Input: part model. Units: mm. Frame: model coordinates. Face numbers are marked on the shaded views. A direction names the side the tool comes from. Round coordinates to 2 decimals unless told otherwise and drop trailing zeros. Order: outer loops, then holes, each group sorted by start corner. A loop starts at its lowest first (then second) coordinate and runs counter-clockwise, first axis right, second up.
Item 1: Line query: L1, parallel to X at y = 12, z = -32; L2, parallel to Z at x = 20, y = 5.5; L3, parallel to Z at x = 37, y = 15. Output: solid intervals per line, ascending.
Item 2: Cut plane A-A on z = -32. Give the number of separate pieces and of enclosed holes in the cut face, then the cut area to 3 significant figures.
Item 3: Cut plane C-C on x = 20. Output: boundary loops of the cut face in (y, z).
Item 4: Cut plane D-D on z = -21. Output: boundary loops of the cut face in (x, y).
Item 5: Reachability of the marked faces 1, 2, 3 and 4 from +Z, -Z, +X, -X, +Y, -Y: full face, straight path, thin tool, end or side. Return the list, or none.
Item 6: Mould query, pull axis X, two halves, no side actions, for the marked faces 5, 6 and 7. Classes: released by +X, released by -X, zero draft, split by the parting line, or undercut.
Item 7: Cut plane B-B on y = 7.25. Output: boundary loops of the cut face in (x, z), then the cut area to 3 significant figures.
Item 8: First-contact query: pin 1 (5 mm diameter, centred on x = 4.5, z = -32, fed in from +Y); pin 2 (1 mm diameter, centred on y = 26.5, z = -12, fed in from +X); pin 3 (3.5 mm diameter, centred on y = 24, z = -7, fed in from -X). Flat tips, straight axial feed; report the tip coordinate or a pass-through.
```python
from build123d import *

# Parameters (mm, degrees)
ESBO_O2_W                = 40
ESBO_O2_H                = 45
CORPO_DEPTH              = 20
ESBO_O3_R                = 12
ESBO_O3_W                = 17.5
ESBO_O3_H                = 9
ENCAIXE_DO_MOTOR_DEPTH   = 19
ESBO_O5_R                = 1.5
CORTE_EXTRUS_O2_DEPTH    = 64.442887702
ESBO_O6_W                = 6.5
ESBO_O6_H                = 5
CORTE_EXTRUS_O3_DEPTH    = 64.442887702
ESBO_O7_W                = 9
ESBO_O7_H                = 21.613382206
CORTE_EXTRUS_O4_DEPTH    = 5
ESBO_O8_W                = 7
ESBO_O8_H                = 7
RESSALTO_EXTRUS_O2_DEPTH = 10


with BuildPart() as part:
    # Esboço2 → Corpo (new body)
    with BuildSketch(Plane(origin=(0, 0, 0), x_dir=(1, 0, 0), z_dir=(0, 1, 0))):
        with Locations((20, 22.5)):
            Rectangle(ESBO_O2_W, ESBO_O2_H)
    extrude(amount=CORPO_DEPTH)

    # Esboço3 → Encaixe do Motor (cut)
    with BuildSketch(Plane(origin=(0, 20, 0), x_dir=(1, 0, 0), z_dir=(0, 1, 0))):
        with Locations((20, 32)):
            Circle(ESBO_O3_R)
        with Locations((20, 20)):
            Rectangle(ESBO_O3_W, ESBO_O3_H)
    extrude(amount=-ENCAIXE_DO_MOTOR_DEPTH, mode=Mode.SUBTRACT)

    # Esboço5 → Corte-extrusão2 (cut, through all)
    with BuildSketch(Plane(origin=(0, 20, 0), x_dir=(1, 0, 0), z_dir=(0, 1, 0))):
        with Locations(Location((4.5, 32, 0), (0, 0, 270))):
            Circle(ESBO_O5_R)
        with Locations(Location((35.5, 32, 0), (0, 0, 270))):
            Circle(ESBO_O5_R)
    extrude(amount=-CORTE_EXTRUS_O2_DEPTH, mode=Mode.SUBTRACT)

    # Esboço6 → Corte-extrusão3 (cut, through all)
    with BuildSketch(Plane(origin=(40, 0, 0), x_dir=(0, 0, -1), z_dir=(1, 0, 0))):
        with Locations((32, 15)):
            Rectangle(ESBO_O6_W, ESBO_O6_H)
    extrude(amount=-CORTE_EXTRUS_O3_DEPTH, mode=Mode.SUBTRACT)

    # Esboço7 → Corte-extrusão4 (cut)
    with BuildSketch(Plane(origin=(0, 20, 0), x_dir=(1, 0, 0), z_dir=(0, 1, 0))):
        with Locations((20, 7.545181244)):
            Rectangle(ESBO_O7_W, ESBO_O7_H)
    extrude(amount=-CORTE_EXTRUS_O4_DEPTH, mode=Mode.SUBTRACT)

    # Esboço8 → Ressalto-extrusão2 (add)
    with BuildSketch(Plane(origin=(0, 20, 0), x_dir=(1, 0, 0), z_dir=(0, 1, 0))):
        with Locations((32.5, 7.5)):
            Rectangle(ESBO_O8_W, ESBO_O8_H)
        with Locations((7.5, 7.5)):
            Rectangle(ESBO_O8_W, ESBO_O8_H)
    extrude(amount=RESSALTO_EXTRUS_O2_DEPTH)


solid = part.part
```
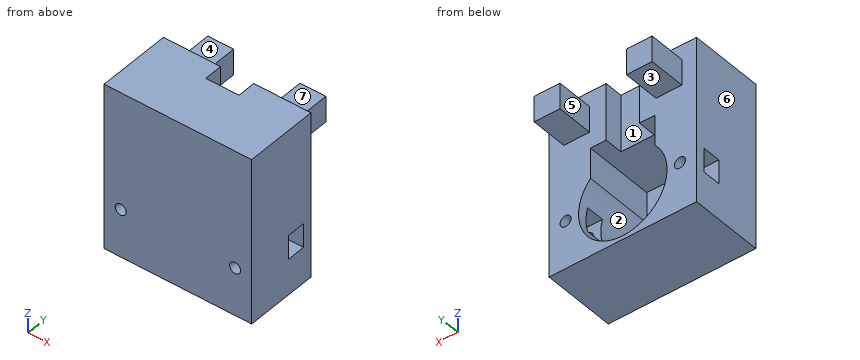
From the geometry:
1. L1: x = 0 to 3, 6 to 8, 32 to 34, 37 to 40
1. L2: z = -45 to -44, -15.5 to 0
1. L3: z = -45 to -35.25, -28.75 to 0
2. separate pieces: 7
2. enclosed holes: 0
2. area: 174 mm2
3. outline: (0, -45) - (20, -45) - (20, -44) - (1, -44) - (1, -15.5) - (15, -15.5) - (15, 0) - (0, 0) - close
4. outline: (0, 0) - (40, 0) - (40, 20) - (28.75, 20) - (28.75, 1) - (11.25, 1) - (11.25, 20) - (0, 20) - close
5. face 1: +Z, +Y
5. face 2: +Y
5. face 3: -Z, +X, -X, +Y
5. face 4: +Z, +X, -X, +Y
6. face 5: undercut
6. face 6: released by -X
6. face 7: zero draft
7. outline: (0, -45) - (40, -45) - (40, 0) - (0, 0) - close; hole circle Ø3 at (4.5, -32); hole (11.25, -23.79) arc R12 ccw (long way) to (28.75, -23.79) - (28.75, -15.5) - (11.25, -15.5) - close; hole circle Ø3 at (35.5, -32)
7. area: 1,230 mm2
8. pin 1: stops at y = 20
8. pin 2: passes through
8. pin 3: stops at x = 4
